CAD build for the part. Positions are in the model's coordinates, mm. A direction names the side the tool comes from. Round coordinates to 2 decimals unless told otherwise and drop trailing zeros. Order: outer loops, then holes, each group sorted by start corner. A loop starts at its lowest first (then second) coordinate and runs counter-clockwise, first axis right, second up. Notation, with made-up numbers: M 87,64 L 127,64 A30 cw 127,97 Z; hole C 1,65 d10. An arc over 180 degrees is marked long. Answer as a JSON object with one key per item and string values. Group by question number.
```python
from build123d import *

# Parameters (mm, degrees)
BOSS_EXTRUDE1_DEPTH = 9.6
FILLET1_R           = 4.8
SKETCH2_R           = 2.3
CUT_EXTRUDE1_DEPTH  = 10


with BuildPart() as part:
    # Sketch1 → Boss-Extrude1 (new body)
    with BuildSketch(Plane.XY):
        with BuildLine():
            ThreePointArc((3.85, 0), (-2.722361108, 2.722361108), (0, -3.85))
            Line((0, -3.85), (15.15, -3.85))
            Line((15.15, -3.85), (15.15, -2.45))
            Line((15.15, -2.45), (2.969848481, -2.45))
            Line((2.969848481, -2.45), (0.084155525, -2.498583168))
            ThreePointArc((0.084155525, -2.498583168), (0.042083726, -2.499645767), (0, -2.5))
            ThreePointArc((0, -2.5), (-1.767766953, 1.767766953), (2.5, 0))
            ThreePointArc((2.5, 0), (2.390405697, -0.732093302), (2.071231518, -1.4))
            Line((2.071231518, -1.4), (15.15, -1.4))
            Line((15.15, -1.4), (15.15, 0))
            Line((15.15, 0), (3.85, 0))
        make_face()
    extrude(amount=BOSS_EXTRUDE1_DEPTH)

    # Fillet1
    fillet1_edges = [part.edges().sort_by_distance(p)[0] for p in [
        (15.15, -0.7, 0),
        (15.15, -0.7, 9.6),
        (15.15, -3.15, 0),
        (15.15, -3.15, 9.6),
    ]]
    fillet(fillet1_edges, radius=FILLET1_R - 0.0001)  # a hair under: the kernel refuses the full size

    # Sketch2 → Cut-Extrude1 (cut)
    with BuildSketch(Plane(origin=(0, 0, 0), x_dir=(1, 0, 0), z_dir=(0, 1, 0))):
        with Locations(Location((10.35, -4.8, 0), (0, 0, 180))):
            Circle(SKETCH2_R)
    extrude(amount=-CUT_EXTRUDE1_DEPTH, mode=Mode.SUBTRACT)


solid = part.part
```
Item 1: Drill centre lines: line 1 (Y direction, x = 5, z = 5); line 2 (Z direction, x = 10.35, y = -0.9). Where is each one in solid material? Low to high. Write a range as [from, to].
Item 2: Cut at A-A, the plane x = 4.25. Give the cut face in (y, z).
Item 3: Cut at B-B, the plane y = -0.5. Give the number of separate pieces and of enclosed holes in the cut face, and give its area (3 significant figures).
Item 4: Flat gauge pins, fed straight in: pin 1 Ø1.5 at (x, z) = (13, 4) entering from +Y; pin 2 Ø1.5 at (y, z) = (0, 6.5) entering from +X; pin 3 Ø1.5 at (x, z) = (-1, 7.5) entering from +Y. Where does each tip first touch, or does it go through?
Item 5: Cut at C-C, the plane x = 9. Give the cut face in (y, z), and give its area (3 significant figures).
Item 6: Two-plate mould, pull along X, no slides. Class faces 1 (the face through (6, -3.85, 5)), 2 (the face through (12.648, -0.69, 4.901)), 3 (the face through (13.78, -3.14, 1.44)), 4 (the face through (12.648, -3.14, 4.901)): +X half, -X half, draft (parallel to the pull), parting line (faces both ways), or undercut.
Item 7: 3-axis set-ups, long thin cutter, end or side, ignore diameter. For faces 5 (the face through (8, 0, 4)), 6 (the face through (13.78, -3.14, 8.16)), 7 (the face through (7.8, -2.45, 4.7)): which of +Z, -Z, +X, -X, +Y, -Y reach the whole face in a straight line?
Response values:
{
 "1": {"line 1": "[-3.85, -2.45], [-1.4, 0]", "line 2": "[0, 2.5], [7.1, 9.6]"},
 "2": {"outline": "M -3.85,0 L -2.45,0 L -2.45,9.6 L -3.85,9.6 Z; M -1.4,0 L 0,0 L 0,9.6 L -1.4,9.6 Z"},
 "3": {"separate pieces": "2", "enclosed holes": "1", "area": "109 mm^2"},
 "4": {"pin 1": "y = 0", "pin 2": "x = 15.06", "pin 3": "y = 3.84"},
 "5": {"outline": "M -3.85,0 L -2.45,0 L -2.45,2.94 L -3.85,2.94 Z; M -3.85,6.66 L -2.45,6.66 L -2.45,9.6 L -3.85,9.6 Z; M -1.4,0 L 0,0 L 0,2.94 L -1.4,2.94 Z; M -1.4,6.66 L 0,6.66 L 0,9.6 L -1.4,9.6 Z", "area": "16.5 mm^2"},
 "6": {"face 1": "draft", "face 2": "undercut", "face 3": "+X half", "face 4": "undercut"},
 "7": {"face 5": "+Z, -Z, +X, +Y", "face 6": "+Z, +X, +Y, -Y", "face 7": "+Z, -Z, +X"}
}
